For this review, take the finished solid that the model builds, in its own axes (mm). A direction names the side the tool comes from. Coordinates: 2 decimals unless noted, no trailing zeros. Loops run counter-clockwise (first coordinate to the right, second up) from the corner with the lowest first, then second, coordinate; pieces in that order, holes last.
```python
from build123d import *

# Parameters (mm, degrees)
SKETCH1_R           = 3.048
BOSS_EXTRUDE1_DEPTH = 21.844
SKETCH2_W           = 24.257
SKETCH2_H           = 14.478
CUT_EXTRUDE1_DEPTH  = 20.2565


with BuildPart() as part:
    # Sketch1 → Boss-Extrude1 (new body)
    with BuildSketch(Plane(origin=(0, 0, 0), x_dir=(1, 0, 0), z_dir=(0, 1, 0))):
        Polygon((-28.065439725, 26.112877044), (-20.953014773, 33.224452067), (20.956985152, 33.221947814), (28.068560175, 26.109522863), (28.065439725, -26.112877044), (20.953014773, -33.224452067), (-20.956985152, -33.221947814), (-28.068560175, -26.109522863), align=None)
        with Locations(Location((0.001666466, 27.88919995, 0), (0, 0, 270))):
            Circle(SKETCH1_R, mode=Mode.SUBTRACT)
        with Locations(Location((-0.001666466, -27.88919995, 0), (0, 0, 270))):
            Circle(SKETCH1_R, mode=Mode.SUBTRACT)
    extrude(amount=BOSS_EXTRUDE1_DEPTH)

    # Sketch2 → Cut-Extrude1 (cut)
    with BuildSketch(Plane(origin=(0, 21.844, 0), x_dir=(1, 0, 0), z_dir=(0, 1, 0))):
        with Locations((-0.001985189, -26.238199941)):
            Rectangle(SKETCH2_W, SKETCH2_H)
        with Locations((-0.001985189, 26.238168907)):
            Rectangle(SKETCH2_W, SKETCH2_H)
    extrude(amount=-CUT_EXTRUDE1_DEPTH, mode=Mode.SUBTRACT)


solid = part.part
```
Q1. Consider section B-B (x = 1). State the section outline as (y, z) points.
Q2. Consider section C-C (y = 12.5). State the section outline as (x, z) points.
Q3. The part is to be moulded in two halves that separate along Z. For faces 4 (the face through (0, 12, -18.999)), 5 (the face through (0.917, 0.783, -24.982)), 6 (the face through (0.132, 0.783, 24.844)), 7 (the face through (0, 0, 0)), say which applies: +Z half, -Z half, draft (parallel to the pull), parting line (faces both ways), or undercut.
Q4. Consider section A-A (z = 28). State the section outline as (x, y) points, then the cut area to 3 significant figures.
Q5. Machinability: for faces 1 (the face through (-24.46, 10.77, 29.72)), 2 (the face through (-0.2, 1.588, -24.6)), 3 (the face through (0, 12, 18.999)), which of the approach directions +Z, -Z, +X, -X, +Y, -Y give a long, thin tool a straight path to every point of the face, cutting with its end or side? Answer none if there is none.
Q6. For pin 1 Ø4.5 at (y, z) = (15.5, -29) entering from -X; pin 2 Ø4 at (x, y) = (-7.5, 4.5) entering from +Z; pin 3 Ø3 at (y, z) = (16, -23) entering from -X, all flat-tipped, find the tip position at first contact; note any pin that passes through.
Q7. Consider section D-D (x = 24). State the section outline as (y, z) points.
Q8. Wall thickness on probe 1 along X at (y, z) = (15, 20); probe 2 along Z at (x, y) = (-14.5, 5); probe 3 along X at (y, z) = (14.5, 0): over which ranges is each line inside the solid? List them lowest first.
Model answer:
1. outline: (0, -33.22) - (1.59, -33.22) - (1.59, -30.77) - (0, -30.77) - close; (0, -25.01) - (1.59, -25.01) - (1.59, -19) - (21.84, -19) - (21.84, 19) - (1.59, 19) - (1.59, 25.01) - (0, 25.01) - close; (0, 30.77) - (1.59, 30.77) - (1.59, 33.22) - (0, 33.22) - close
2. outline: (-28.07, -26.11) - (-20.95, -33.22) - (-12.13, -33.22) - (-12.13, -19) - (12.13, -19) - (12.13, -33.22) - (20.96, -33.22) - (28.07, -26.11) - (28.07, 26.11) - (20.95, 33.22) - (12.13, 33.22) - (12.13, 19) - (-12.13, 19) - (-12.13, 33.22) - (-20.96, 33.22) - (-28.07, 26.11) - close
3. face 4: -Z half
3. face 5: undercut
3. face 6: undercut
3. face 7: draft
4. outline: (-26.18, 0) - (-3.05, 0) - (-3.05, 1.59) - (-12.13, 1.59) - (-12.13, 21.84) - (-26.18, 21.84) - close; (3.04, 0) - (26.18, 0) - (26.18, 21.84) - (12.13, 21.84) - (12.13, 1.59) - (3.04, 1.59) - close
4. area: 643 mm2
5. face 1: +Z, -X, +Y, -Y
5. face 2: -Z, +Y
5. face 3: +Z, +Y
6. pin 1: stops at x = -27.43
6. pin 2: stops at z = 19
6. pin 3: stops at x = -28.07
7. outline: (0, -30.18) - (21.84, -30.18) - (21.84, 30.18) - (0, 30.18) - close
8. probe 1: x = -28.07 to -12.13, 12.13 to 28.07
8. probe 2: z = -33.22 to 33.22
8. probe 3: x = -28.07 to 28.07
